For this review, take the finished solid that the model builds, in its own axes (mm). A direction names the side the tool comes from. Round coordinates to 2 decimals unless told otherwise and drop trailing zeros. Write each loop counter-clockwise with the first axis right and the second up, starting at its lowest first coordinate (ties: lowest second). Pieces come first, ordered by that corner, then holes. Notation, with made-up numbers: M 39,55.5 L 96,55.5 A15 cw 96,60.5 Z; hole C 10.25,-26 d8. An arc over 180 degrees is marked long. Answer in a Markdown table with one row per item.
```python
from build123d import *

# Parameters (mm, degrees)
SKETCH1_W           = 25
SKETCH1_H           = 15
BOSS_EXTRUDE1_DEPTH = 30
FILLET1_R           = 2
SHELL1_START        = -10.5
SHELL1_OUTLINE_W    = 30
SHELL1_OUTLINE_H    = 10
SHELL1_DEPTH        = 21
FILLET3_R           = 1


# Read off the part's stored shape, not the designer's step: Shell1
with BuildPart() as part:
    # Sketch1 → Boss-Extrude1 (new body)
    with BuildSketch(Plane(origin=(0, 0, 0), x_dir=(0, 0, -1), z_dir=(1, 0, 0))):
        Rectangle(SKETCH1_W, SKETCH1_H)
    extrude(amount=BOSS_EXTRUDE1_DEPTH)

    # Fillet1
    fillet1_edges = [part.edges().sort_by_distance(p)[0] for p in [
        (15, -7.5, -12.5),
        (15, -7.5, 12.5),
        (15, 7.5, 12.5),
        (15, 7.5, -12.5),
    ]]
    fillet(fillet1_edges, radius=FILLET1_R)

    # Shell1 outline → Shell1 (cut)
    with BuildSketch(Plane.XY.offset(SHELL1_START)):
        with Locations((15, 0.5)):
            Rectangle(SHELL1_OUTLINE_W, SHELL1_OUTLINE_H)
    extrude(amount=SHELL1_DEPTH, mode=Mode.SUBTRACT)

    # Fillet3
    fillet3_edges = [part.edges().sort_by_distance(p)[0] for p in [
        (15, 5.5, -10.5),
        (15, 5.5, 10.5),
        (15, -4.5, 10.5),
        (15, -4.5, -10.5),
    ]]
    fillet(fillet3_edges, radius=FILLET3_R)


solid = part.part
```
Q1. For probe 1 along Z at (x, y) = (25, 4.5); probe 2 along Y at (x, z) = (26, -8); probe 3 along Z at (x, y) = (4.5, 5), list the stretches that pass through material, from the lowest coordinate up.
Found:
| item | result |
|---|---|
| probe 1 | -12.5 to -10.5, 10.5 to 12.5 |
| probe 2 | -7.5 to -4.5, 5.5 to 7.5 |
| probe 3 | -12.5 to -10.37, 10.37 to 12.5 |
Q2. Take a section at A-A (z = 5). State the section outline as (x, y) points.
Found:
| item | result |
|---|---|
| outline | M 0,-7.5 L 30,-7.5 L 30,-4.5 L 0,-4.5 Z; M 0,5.5 L 30,5.5 L 30,7.5 L 0,7.5 Z |
Q3. Mouldability with a two-part tool opening along Y and no side actions: class faces 1 (the face through (15.21, -4.199, 10.215)), 2 (the face through (15, -7.5, 0)), 3 (the face through (15.21, 6.9, 11.93)) as +Y half, -Y half, draft (parallel to the pull), parting line (faces both ways), or undercut.
Found:
| item | result |
|---|---|
| face 1 | undercut |
| face 2 | -Y half |
| face 3 | +Y half |
Q4. Take a section at D-D (y = -6.5). State the section outline as (x, z) points.
Found:
| item | result |
|---|---|
| outline | M 0,-12.23 L 30,-12.23 L 30,12.23 L 0,12.23 Z |
Q5. Take a section at C-C (y = 3.75). State the section outline as (x, z) points.
Found:
| item | result |
|---|---|
| outline | M 0,-12.5 L 30,-12.5 L 30,-10.5 L 0,-10.5 Z; M 0,10.5 L 30,10.5 L 30,12.5 L 0,12.5 Z |
Q6. Take a section at B-B (x = 13.5). State the section outline as (y, z) points.
Found:
| item | result |
|---|---|
| outline | M -7.5,-10.5 A2 ccw -5.5,-12.5 L 5.5,-12.5 A2 ccw 7.5,-10.5 L 7.5,10.5 A2 ccw 5.5,12.5 L -5.5,12.5 A2 ccw -7.5,10.5 Z; hole M -4.5,-9.5 A1 ccw -3.5,-10.5 L 4.5,-10.5 A1 ccw 5.5,-9.5 L 5.5,9.5 A1 ccw 4.5,10.5 L -3.5,10.5 A1 ccw -4.5,9.5 Z |
Q7. Machinability: for faces 4 (the face through (15.21, 5.215, 10.199)), 5 (the face through (15.21, -6.93, -11.9)), which of the approach directions +Z, -Z, +X, -X, +Y, -Y give a long, thin tool a straight path to every point of the face, cutting with its end or side? Answer none if there is none.
Found:
| item | result |
|---|---|
| face 4 | +X, -X |
| face 5 | -Z, +X, -X, -Y |
